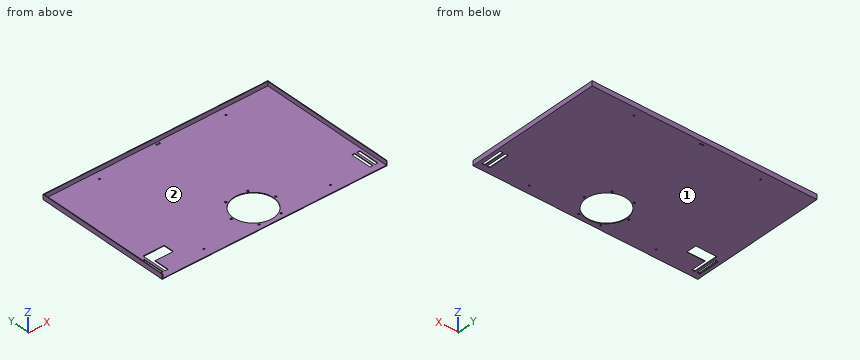
```python
from build123d import *

# Parameters (mm, degrees)
F0_R     = 3.5
F0_R_2   = 4.5
F0_R_3   = 95
F0_W     = 14
F0_H     = 30
F1_DEPTH = 3
F3_DEPTH = 20
F4_W     = 14
F4_H     = 70
F4_H_2   = 100
F5_DEPTH = 3.001


with BuildPart() as f1:
    # F0 (on Top) → F1 (new body)
    with BuildSketch(Plane.XY):
        Polygon((533, -325), (533, 325), (-533, 325), (-533, -325), (-517, -325), (-517, -295), (-517, -195), (-503, -195), (-503, -295), (-503, -325), (503, -325), (503, -295), (503, -195), (517, -195), (517, -295), (517, -325), align=None)
        with Locations((-300, -285)):
            Circle(F0_R, mode=Mode.SUBTRACT)
        Polygon((-493, -175), (-468, -175), (-418, -175), (-393, -175), (-393, -225), (-418, -225), (-468, -225), (-493, -225), align=None, mode=Mode.SUBTRACT)
        with Locations((-52.5, -300.932667)):
            Circle(F0_R_2, mode=Mode.SUBTRACT)
        with Locations((-105, -210)):
            Circle(F0_R_2, mode=Mode.SUBTRACT)
        with Locations((-52.5, -119.067333)):
            Circle(F0_R_2, mode=Mode.SUBTRACT)
        with Locations((52.5, -300.932667)):
            Circle(F0_R_2, mode=Mode.SUBTRACT)
        with Locations((0, -210)):
            Circle(F0_R_3, mode=Mode.SUBTRACT)
        with Locations((105, -210)):
            Circle(F0_R_2, mode=Mode.SUBTRACT)
        with Locations((300, -285)):
            Circle(F0_R, mode=Mode.SUBTRACT)
        with Locations((52.5, -119.067333)):
            Circle(F0_R_2, mode=Mode.SUBTRACT)
        with Locations((-300, 285)):
            Circle(F0_R, mode=Mode.SUBTRACT)
        with Locations((-6, 310)):
            Circle(F0_R, mode=Mode.SUBTRACT)
        with Locations((6, 310)):
            Circle(F0_R, mode=Mode.SUBTRACT)
        with Locations((300, 285)):
            Circle(F0_R, mode=Mode.SUBTRACT)
        with Locations((-510, -310)):
            Rectangle(F0_W, F0_H)
        with Locations((510, -310)):
            Rectangle(F0_W, F0_H)
    extrude(amount=-F1_DEPTH)

    # F2 (on face) → F3 (join)
    with BuildSketch(Plane.XY):
        Polygon((-533, -325), (-530, -325), (-530, 322), (530, 322), (530, -325), (533, -325), (533, 325), (-533, 325), align=None)
    extrude(amount=F3_DEPTH)

    # F4 (on face) → F5 (cut, through all)
    with BuildSketch(Plane.XY):
        with Locations((-486, -260)):
            Rectangle(F4_W, F4_H)
        with Locations((486, -245)):
            Rectangle(F4_W, F4_H_2)
    extrude(amount=-F5_DEPTH, mode=Mode.SUBTRACT)


solid = f1.part
```
The listing builds one solid part. Answer for the finished solid, in the listing's coordinates (mm). Face numbers are marked on the shaded views. Give positions to 0.01 mm unless a question says otherwise; leave off trailing zeros. Order: outer loops, then holes, each group sorted by start corner. A loop starts at its lowest first (then second) coordinate and runs counter-clockwise, first axis right, second up. Notation, with made-up numbers: (-28.5, -17.5) -> (15.5, -17.5) arc R29 ccw to (15.5, 13.5) -> close; hole circle Ø6 at (-3.5, 51). An arc over 180 degrees is marked (long way). Write each question's results on one line, items separated by ' | '.
Q1. Determine the mould class of the marked faces 1 and 2 for opening direction X: pulls with the +X half, pulls with the -X half, needs draft (parallel to the pull), parting line crosses it, or undercut.
Checked values:
face 1: needs draft | face 2: undercut
Q2. Straight lines are drawn through the part: probe 1 along X at (y, z) = (285, -0.7); probe 2 along Y at (x, z) = (300, -1); probe 3 along Y at (x, z) = (6, -1.25). For each, find the intervals that lie inside material, in ascending order. Write a range as from..to.
Checked values:
probe 1: x = -533..-303.5, -296.5..296.5, 303.5..533 | probe 2: y = -325..-288.5, -281.5..281.5, 288.5..325 | probe 3: y = -325..-304.81, -115.19..306.5, 313.5..325
Q3. Each of these flat-tipped pins is pushed along its axis until it touches: P1, Ø9, axis at x = 6, y = 310, coming from the +Z side; P2, Ø1, axis at x = 171, z = 7.5, coming from the -Y side. Where does it stop, or does it pass through?
Checked values:
P1: stops at z = 0 | P2: stops at y = 322
Q4. The part is cut by section B-B, the plane y = -143.5. Give the vertices of the cut face in (x, z).
Checked values:
outline: (-533, -3) -> (-67.84, -3) -> (-67.84, 0) -> (-530, 0) -> (-530, 20) -> (-533, 20) -> close; (67.84, -3) -> (533, -3) -> (533, 20) -> (530, 20) -> (530, 0) -> (67.84, 0) -> close
Q5. The part is cut by section D-D, the plane y = 218.5. Give the vertices of the cut face in (x, z), and give its area (3 significant figures).
Checked values:
outline: (-533, -3) -> (533, -3) -> (533, 20) -> (530, 20) -> (530, 0) -> (-530, 0) -> (-530, 20) -> (-533, 20) -> close | area: 3,320 mm^2
Q6. The part is cut by section C-C, the plane x = 346.5. Give the vertices of the cut face in (y, z).
Checked values:
outline: (-325, -3) -> (325, -3) -> (325, 20) -> (322, 20) -> (322, 0) -> (-325, 0) -> close
Q7. The part is cut by section A-A, the plane z = 10.5. Give the vertices of the cut face in (x, y), and give its area (3 significant figures).
Checked values:
outline: (-533, -325) -> (-530, -325) -> (-530, 322) -> (530, 322) -> (530, -325) -> (533, -325) -> (533, 325) -> (-533, 325) -> close | area: 7,080 mm^2
